```python
from build123d import *

# Parameters (mm, degrees)
CROQUIS1_W                = 50.8
CROQUIS1_H                = 50.8
SALIENTE_EXTRUIR1_DEPTH   = 100
SALIENTE_EXTRUIR1_2_DEPTH = 100
SALIENTE_EXTRUIR1_3_DEPTH = 100
SALIENTE_EXTRUIR1_4_DEPTH = 100
SALIENTE_EXTRUIR2_REACH   = 390.458
CROQUIS2_W                = 280
CROQUIS2_H                = 12.7


with BuildPart() as part:
    # Croquis1 → Saliente-Extruir1 (new body)
    with BuildSketch(Plane(origin=(0, 0, 0), x_dir=(1, 0, 0), z_dir=(0, 1, 0))):
        with Locations((25.4, -25.4)):
            Rectangle(CROQUIS1_W, CROQUIS1_H)
    extrude(amount=SALIENTE_EXTRUIR1_DEPTH)


with BuildPart() as body_2:
    # Croquis1 → Saliente-Extruir1 2 (new body)
    with BuildSketch(Plane(origin=(0, 0, 0), x_dir=(1, 0, 0), z_dir=(0, 1, 0))):
        with Locations((254.6, -25.4)):
            Rectangle(CROQUIS1_W, CROQUIS1_H)
    extrude(amount=SALIENTE_EXTRUIR1_2_DEPTH)

    # Saliente-Extruir2: up to this face of the body (flat: up to its plane)
    saliente_extruir2_end = Plane(body_2.part.faces().sort_by_distance((254.6, 50, 0))[0])
    # Croquis2 → Saliente-Extruir2 (add, up to the picked face)
    with BuildSketch(Plane.XY.offset(250), mode=Mode.PRIVATE) as saliente_extruir2_sk1:
        with Locations((140, 93.65)):
            Rectangle(CROQUIS2_W, CROQUIS2_H)
    saliente_extruir2_tool1 = split(extrude(saliente_extruir2_sk1.sketch, amount=-SALIENTE_EXTRUIR2_REACH, mode=Mode.PRIVATE), bisect_by=saliente_extruir2_end, keep=Keep.BOTH, mode=Mode.PRIVATE)

    add(part.part)  # Saliente-Extruir2 merges part


with BuildPart() as body_3:
    # Croquis1 → Saliente-Extruir1 3 (new body)
    with BuildSketch(Plane(origin=(0, 0, 0), x_dir=(1, 0, 0), z_dir=(0, 1, 0))):
        with Locations((254.6, -224.6)):
            Rectangle(CROQUIS1_W, CROQUIS1_H)
    extrude(amount=SALIENTE_EXTRUIR1_3_DEPTH)


with BuildPart() as body_4:
    # Croquis1 → Saliente-Extruir1 4 (new body)
    with BuildSketch(Plane(origin=(0, 0, 0), x_dir=(1, 0, 0), z_dir=(0, 1, 0))):
        with Locations((25.4, -224.6)):
            Rectangle(CROQUIS1_W, CROQUIS1_H)
    extrude(amount=SALIENTE_EXTRUIR1_4_DEPTH)


with BuildPart() as body_2_1:
    add(body_2.part)

    add(body_3.part)  # Saliente-Extruir2 merges body 3

    add(body_4.part)  # Saliente-Extruir2 merges body 4
    add(saliente_extruir2_tool1.solids().sort_by(Axis((140, 93.65, 250), (0, 0, -1)))[0])


solid = body_2_1.part
```
Input: part model. Units: mm. Frame: model coordinates. A direction names the side the tool comes from. Give positions to 0.01 mm unless a question says otherwise; leave off trailing zeros. Loops run counter-clockwise (first coordinate to the right, second up) from the corner with the lowest first, then second, coordinate; pieces in that order, holes last. Notation, with made-up numbers: M 8.5,29 L 34.5,29 A28 cw 34.5,58 Z; hole C 13.25,64 d7. An arc over 180 degrees is marked long. Answer as CSV lines item,"result". Start each with the question number.
1. Section A-A on y = 59. Return loops of the section in (x, z), plus the area to 3 significant figures.
2. Section B-B on x = 32. Return loops of the section in (y, z).
3. Section D-D on x = 73. Return loops of the section in (y, z), plus the area to 4 significant figures.
4. Pull-direction query (X, two-part tool) for faces 4 (the face through (280, 94, 127)), 5 (the face through (229.2, 43, 26)), 6 (the face through (25, 43, 199.2)); classes: released by +X, released by -X, zero draft, split by the parting line, or undercut.
5. Reachability of faces 1 (the face through (138, 94, 0)), 2 (the face through (25, 43, 50.8)), 3 (the face through (50.8, 43, 225)) from +Z, -Z, +X, -X, +Y, -Y: full face, straight path, thin tool, end or side. Return the list, or none.
6. Section C-C on z = 73. Return loops of the section in (x, y).
7. Line query: L1, parallel to X at y = 75, z = 233; L2, parallel to Y at x = 135, z = 94; L3, parallel to Z at x = 246, y = 22.5. Output: solid intervals per line, ascending.
8. Pin query (flat end, axial travel): P1, Ø10, axis at x = 242, y = 66, coming from the -Z side. Return the tip coordinate at first contact, or that it passes through.
Computed values:
1,outline,"M 0,0 L 50.8,0 L 50.8,50.8 L 0,50.8 Z; M 0,199.2 L 50.8,199.2 L 50.8,250 L 0,250 Z; M 229.2,0 L 280,0 L 280,50.8 L 229.2,50.8 Z; M 229.2,199.2 L 280,199.2 L 280,250 L 229.2,250 Z"
1,area,"10,300 mm²"
2,outline,"M 0,0 L 100,0 L 100,250 L 0,250 L 0,199.2 L 87.3,199.2 L 87.3,50.8 L 0,50.8 Z"
3,outline,"M 87.3,0 L 100,0 L 100,250 L 87.3,250 Z"
3,area,"3,175 mm²"
4,face 4,"released by +X"
4,face 5,"undercut"
4,face 6,"zero draft"
5,face 1,"-Z, +X, -X, +Y, -Y"
5,face 2,"+X, -X, -Y"
5,face 3,"+Z, -Z, -Y"
6,outline,"M 0,87.3 L 280,87.3 L 280,100 L 0,100 Z"
7,L1,"x = 0 to 50.8, 229.2 to 280"
7,L2,"y = 87.3 to 100"
7,L3,"z = 0 to 50.8, 199.2 to 250"
8,P1,"stops at z = 0"
